Can you work these out from the model? Positions are in its coordinate system, mm. Face numbers are marked on the shaded views. Round coordinates to 2 decimals unless told otherwise and drop trailing zeros. Write each loop counter-clockwise with the first axis right and the second up, starting at its lowest first coordinate (ties: lowest second). Pieces come first, ordered by that corner, then holes.
Q1. If we section it at A-A (z = 25): Please give me the cut outline in (x, y), plus the area to 3 significant figures.
Q2. I'm going to push a flat-ended pin straight in: pin 1 Ø4 at (x, y) = (-10, 22) entering from +Z. Where does the tip first touch, or does it pass through?
Q3. If we section it at D-D (z = 34.5): Please give me the cut outline in (x, y), plus the area to 3 significant figures.
Q4. We'd pull the mould along X, two halves only. Please class the marked faces 1, 2 and 3: +X half, -X half, draft (parallel to the pull), parting line (faces both ways), or undercut.
Q5. If we section it at B-B (y = -7.5): Please give me the cut outline in (x, z), plus the area to 3 significant figures.
Q6. If we section it at C-C (x = 0): Please give me the cut outline in (y, z), plus the area to 3 significant figures.
Q7. Please list where these lines run through material, in increasing order: line 1 along X through (y, z) = (28.5, 25); line 2 along X through (y, z) = (8, 35.5); line 3 along Z through (x, y) = (0, -17).
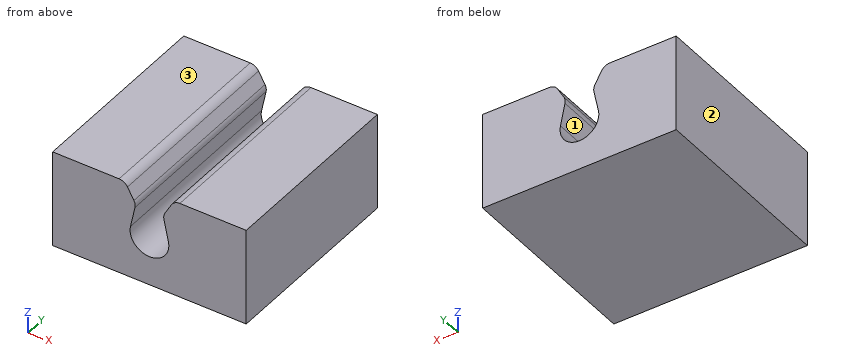
from build123d import *

# Parameters (mm, degrees)
SKIZZE1_W                       = 100
SKIZZE1_H                       = 100
AUFSATZ_LINEAR_AUSTRAGEN1_DEPTH = 50
SCHNITT_LINEAR_AUSTRAGEN1_DEPTH = 101
VERRUNDUNG1_R                   = 5


with BuildPart() as part:
    # Skizze1 → Aufsatz-Linear austragen1 (new body)
    with BuildSketch(Plane.XY):
        Rectangle(SKIZZE1_W, SKIZZE1_H)
    extrude(amount=AUFSATZ_LINEAR_AUSTRAGEN1_DEPTH)

    # Skizze2 → Schnitt-Linear austragen1 (cut, through all)
    with BuildSketch(Plane.XZ.offset(50)):
        with BuildLine():
            ThreePointArc((-9.789261077, 27.042147785), (0, 15), (9.789261077, 27.042147785))
            Line((9.789261077, 27.042147785), (7.086110247, 40))
            Line((7.086110247, 40), (12.79015, 50))
            Line((12.79015, 50), (-12.79015, 50))
            Line((-12.79015, 50), (-7.086110247, 40))
            Line((-7.086110247, 40), (-9.789261077, 27.042147785))
        make_face()
    extrude(amount=-SCHNITT_LINEAR_AUSTRAGEN1_DEPTH, mode=Mode.SUBTRACT)

    # Verrundung1
    verrundung1_edges = [part.edges().sort_by_distance(p)[0] for p in [
        (-12.79015, 0, 50),
        (12.79015, 0, 50),
        (7.086110247, 0, 40),
        (-7.086110247, 0, 40),
    ]]
    fillet(verrundung1_edges, radius=VERRUNDUNG1_R)


solid = part.part
A:
1. outline: (-50, -50) - (-10, -50) - (-10, 50) - (-50, 50) - close; (10, -50) - (50, -50) - (50, 50) - (10, 50) - close
1. area: 8,000 mm2
2. pin 1: stops at z = 48.37
3. outline: (-50, -50) - (-8.23, -50) - (-8.23, 50) - (-50, 50) - close; (8.23, -50) - (50, -50) - (50, 50) - (8.23, 50) - close
3. area: 8,350 mm2
4. face 1: undercut
4. face 2: -X half
4. face 3: draft
5. outline: (-50, 0) - (50, 0) - (50, 50) - (15.69, 50) arc R5 ccw to (11.35, 47.48) - (8.02, 41.64) arc R5 ccw to (7.47, 38.15) - (9.79, 27.04) arc R10 cw (long way) to (-9.79, 27.04) - (-7.47, 38.15) arc R5 ccw to (-8.02, 41.64) - (-11.35, 47.48) arc R5 ccw to (-15.69, 50) - (-50, 50) - close
5. area: 4,380 mm2
6. outline: (-50, 0) - (50, 0) - (50, 15) - (-50, 15) - close
6. area: 1,500 mm2
7. line 1: x = -50 to -10, 10 to 50
7. line 2: x = -50 to -8.02, 8.02 to 50
7. line 3: z = 0 to 15
